```python
from build123d import *


with BuildPart() as f1:
    # F0 (on Front) → F1 (revolve)
    with BuildSketch(Plane.XZ):
        with BuildLine():
            Line((0, 150), (0, 0))
            Line((0, 0), (42.44396, 0))
            ThreePointArc((42.44396, 0), (47.028244, 3.003917), (46.104204, 8.406262))
            Line((46.104204, 8.406262), (22.963254, 33.272674))
            ThreePointArc((22.963254, 33.272674), (21.970476, 34.848801), (21.623498, 36.678936))
            Line((21.623498, 36.678936), (21.623498, 121.950191))
            ThreePointArc((21.623498, 121.950191), (21.540372, 122.858129), (21.293757, 123.735878))
            Line((21.293757, 123.735878), (11.251598, 150))
            Line((11.251598, 150), (0, 150))
        make_face()
    revolve(axis=Axis((0, 0, 75), (0, 0, 1)))


solid = f1.part
```
The listing builds one solid part. Answer for the finished solid, in the listing's coordinates (mm). A direction names the side the tool comes from. Coordinates: 2 decimals unless noted, no trailing zeros. Write each loop counter-clockwise with the first axis right and the second up, starting at its lowest first coordinate (ties: lowest second). Pieces come first, ordered by that corner, then holes. Notation, with made-up numbers: (70.25, -36.75) - (109.25, -36.75) arc R12 ccw to (109.25, -23.75) - close; hole circle Ø1 at (-24, 49). An arc over 180 degrees is marked (long way). Return JSON: item names as keys, results as strings. Group by question number.
Q1. Find the intervals of material crossed by line 1 along Y through (x, z) = (-10, 122); line 2 along X through (y, z) = (13, 34); line 3 along Z through (x, y) = (-39.5, 11), in increasing order. Write a range as [from, to].
Q2. The part is cut by section D-D on z = 19.5. Write down the section's boundary in (x, y), and give its area (3 significant figures).
Q3. Flat-ended cylindrical pins translate along their axes: pin 1 Ø5 at (x, y) = (-0.5, 6) entering from -Z; pin 2 Ø4 at (x, z) = (17.5, 88.5) entering from +Y. Find the tip coordinate at first contact, or state that the pin passes through.
Q4. The part is cut by section A-A on x = 0. Write down the section's boundary in (y, z).
Q5. The part is cut by section C-C on z = 119. Write down the section's boundary in (x, y).
Q6. Which of the six approach directions +Z, -Z, +X, -X, +Y, -Y give full straight-line access (tool end or side, diameter ignored) to faces 1 (the cylindrical face through (9.978, -19.184, 79.911)), 2 (the flat face through (0, 0, 150))?
Evaluation:
{
 "1": {"line 1": "y = [-19.17, 19.17]", "line 2": "x = [-18.24, 18.24]", "line 3": "z = [0, 13.89]"},
 "2": {"outline": "circle Ø71.56 at (0, 0)", "area": "4,020 mm2"},
 "3": {"pin 1": "stops at z = 0", "pin 2": "stops at y = 15.08"},
 "4": {"outline": "(-46.1, 8.41) arc R5 ccw to (-42.44, 0) - (42.44, 0) arc R5 ccw to (46.1, 8.41) - (22.96, 33.27) arc R5 cw to (21.62, 36.68) - (21.62, 121.95) arc R5 ccw to (21.29, 123.74) - (11.25, 150) - (-11.25, 150) - (-21.29, 123.74) arc R5 ccw to (-21.62, 121.95) - (-21.62, 36.68) arc R5 cw to (-22.96, 33.27) - close"},
 "5": {"outline": "circle Ø43.25 at (0, 0)"},
 "6": {"face 1": "+Z", "face 2": "+Z, +X, -X, +Y, -Y"}
}
